Autodesk Inventor part; units mm, degrees
ref_plane "YZ Plane" through (0, 0, 0) normal (1, 0, 0) x (0, 1, 0)
ref_plane "XZ Plane" through (0, 0, 0) normal (0, 1, 0) x (-1, 0, 0)
ref_plane "XY Plane" through (0, 0, 0) normal (0, 0, 1) x (1, 0, 0)
sketch "Sketch1" plane through (0, 0, 0) normal (1, 0, 0) x (0, 1, 0)
  line L0 (6.0697, 14.4062) -> (-19.3303, 14.4062)
  line L1 (-19.3303, 14.4062) -> (-19.3303, -10.9938)
  line L2 (-19.3303, -10.9938) -> (6.0697, -10.9938)
  line L3 (6.0697, -10.9938) -> (6.0697, 14.4062)
  line L4 (2.8947, 11.2312) -> (-16.1553, 11.2312)
  line L5 (-16.1553, 11.2312) -> (-16.1553, -7.8188)
  line L6 (-16.1553, -7.8188) -> (2.8947, -7.8188)
  line L7 (2.8947, -7.8188) -> (2.8947, 11.2312)
  point P0 (0, 0)
  dimension "d0" = 25.4
  dimension "d1" = 25.4
  dimension "d2" = 3.175
extrude "Extrusion1" add sketch "Sketch1" along normal blind 304.8
sketch "Sketch2" plane through (0, 6.0697, 14.4062) normal (0, 1, 0) x (1, 0, 0)
  line L0 (0, 14.4062) -> (12.7, 14.4062)
  line L1 (12.7, 14.4062) -> (38.1, 14.4062)
  circle A0 centre (12.7, 14.4062) radius 2.5797
  circle A1 centre (38.1, 14.4062) radius 2.5797
  line L2 (304.8, 22.225) -> (304.8, 3.175)
  circle A2 centre (139.7096, 14.4062) radius 2.5797
  dimension "d5" = 12.7
  dimension "d6" = 25.4
  dimension "d7" = 5.1594
  dimension "d8" = 5.1594
  dimension "d13" = 5.1594
extrude "Extrusion3" cut sketch "Sketch2" against normal blind 304.8
sketch "Sketch3" plane through (0, 6.0697, 14.4062) normal (0, 1, 0) x (1, 0, 0)
  line L0 (304.8, 3.175) -> (304.8, 22.225)
  line L1 (304.8, 12.7) -> (203.2, 12.7)
  line L2 (0, 25.4) -> (304.8, 25.4)
  line L3 (0, 0) -> (304.8, 0)
  line L4 (203.2, 25.4) -> (304.8, 25.4)
  line L5 (304.8, 25.4) -> (304.8, 0)
  line L6 (304.8, 0) -> (203.2, 0)
  line L7 (203.2, 0) -> (203.2, 25.4)
  point P0 (0, 14.4062)
  dimension "d18" = 101.6
extrude "Extrusion4" cut sketch "Sketch3" against normal blind 304.8
properties part number "Tube Beam"
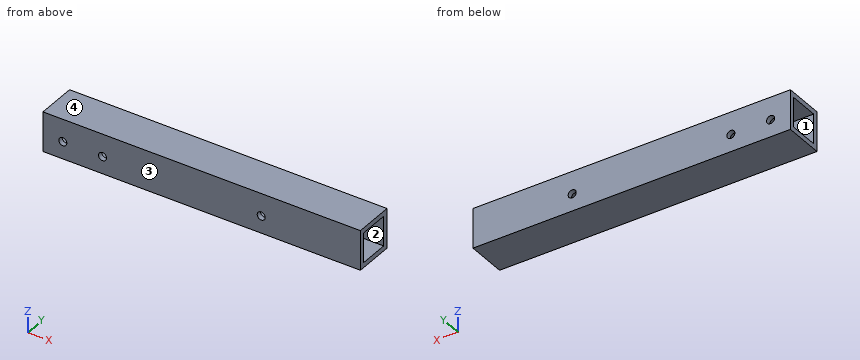
Geometry check sheet. Reference: the model listing, model coordinates, mm. Face numbers are marked on the shaded views. Coordinates: 2 decimals unless noted, no trailing zeros. Write each loop counter-clockwise with the first axis right and the second up, starting at its lowest first coordinate (ties: lowest second). Pieces come first, ordered by that corner, then holes. Notation, with made-up numbers: (28.25, 63) -> (62.25, 63) arc R28 cw to (62.25, 88) -> close; hole circle Ø11 at (29.25, 17). An arc over 180 degrees is marked (long way). One line per question, with ' | ' between items.
1. Cross-section at C-C on x = 38.1. Record the cut outline in (y, z), and give its area (3 significant figures).
Answers:
outline: (-19.33, -10.99) -> (6.07, -10.99) -> (6.07, -2.58) -> (2.89, -2.58) -> (2.89, -7.82) -> (-16.16, -7.82) -> (-16.16, -2.58) -> (-19.33, -2.58) -> close; (-19.33, 2.58) -> (-16.16, 2.58) -> (-16.16, 11.23) -> (2.89, 11.23) -> (2.89, 2.58) -> (6.07, 2.58) -> (6.07, 14.41) -> (-19.33, 14.41) -> close | area: 249 mm²
2. Cross-section at D-D on x = 114.5. Record the cut outline in (y, z), and give its area (3 significant figures).
Answers:
outline: (-19.33, -10.99) -> (6.07, -10.99) -> (6.07, 14.41) -> (-19.33, 14.41) -> close; hole (-16.16, -7.82) -> (2.89, -7.82) -> (2.89, 11.23) -> (-16.16, 11.23) -> close | area: 282 mm²
3. Thickness scan on probe 1 along X at (y, z) = (4.1, 0); probe 2 along Y at (x, z) = (181, 8.75); probe 3 along Z at (x, y) = (137, -7.75). Record the ranges inside material, lowest first. Write a range as from..to.
Answers:
probe 1: x = 0..10.12, 15.28..35.52, 40.68..137.13, 142.29..203.2 | probe 2: y = -19.33..-16.16, 2.89..6.07 | probe 3: z = -10.99..-7.82, 11.23..14.41
4. Cross-section at B-B on y = -14.5. Record the cut outline in (x, z).
Answers:
outline: (0, -10.99) -> (203.2, -10.99) -> (203.2, -7.82) -> (0, -7.82) -> close; (0, 11.23) -> (203.2, 11.23) -> (203.2, 14.41) -> (0, 14.41) -> close
5. Cross-section at A-A on z = 6.5. Record the cut outline in (x, y), and give its area (3 significant figures).
Answers:
outline: (0, -19.33) -> (203.2, -19.33) -> (203.2, -16.16) -> (0, -16.16) -> close; (0, 2.89) -> (203.2, 2.89) -> (203.2, 6.07) -> (0, 6.07) -> close | area: 1,290 mm²
6. Depth check by flat-ended pin: pin 1 Ø2 at (y, z) = (-9, -7.5) entering from -X; pin 2 Ø10 at (y, z) = (-5, 5.5) entering from -X. Enter the tip coordinate at first touch or a pass-through.
Answers:
pin 1: stops at x = 0 | pin 2: passes through
7. Draft check along Z on the marked faces 1, 2, 3 and 4. Enter one of: +Z half, -Z half, draft (parallel to the pull), parting line (faces both ways), or undercut.
Answers:
face 1: undercut | face 2: undercut | face 3: draft | face 4: +Z half
